Build history of the part. All positions in model axes, mm. A direction names the side the tool comes from. Give positions to 0.01 mm unless a question says otherwise; leave off trailing zeros. Write each loop counter-clockwise with the first axis right and the second up, starting at its lowest first coordinate (ties: lowest second). Pieces come first, ordered by that corner, then holes. Notation, with made-up numbers: (87.25, 70) -> (102.25, 70) arc R29 ccw to (102.25, 93) -> close; hole circle Ø8 at (22, 77.5). An arc over 180 degrees is marked (long way). One line per question, with ' | ' between items. Start each with the question number.
(1) Tool access for faces 5 (the flat face through (4.065, 0.801, 2.465)), 6 (the cylindrical face through (4.78, -3.51, 2.46)), 7 (the cylindrical face through (-0.7, 3.3, 2.5)), 8 (the cylindrical face through (-3.014, 1.518, 2.465)), 9 (the cylindrical face through (0.05, 1.65, 2.04)): list every direction of +Z, -Z, +X, -X, +Y, -Y with a clear straight run to the whole face (end or side of a thin tool).
(2) Pull direction X, two halves, no side cores. Call faces 1 (the cylindrical face through (2.19, -5.54, 2.46)), 2 (the flat face through (0, 4, 2)), 3 (the flat face through (-1.2, 2, 5)), 4 (the flat face through (-3.315, -2.486, 2.465)): released by +X, released by -X, zero draft, split by the parting line, or undercut.
(3) Band-saw the part on B-B, the plane x = -5.25. Give the cut face in (y, z), and give its area (3 significant figures).
(4) Band-saw the part on A-A, the plane y = 0. Give the cut face in (x, z) (3 decimals).
(5) Pin check, flat tips, straight feed: P1, Ø1.9, axis at x = 0, z = 3, coming from the +Y side; P2, Ø1.2, axis at y = 4.5, z = 1.5, coming from the -X side; P3, Ø2.5, axis at x = 0, y = 0, coming from the -Z side. Stop position of each tip, or through.
(6) Band-saw the part on D-D, the plane x = 6.5. Give the cut face in (y, z).
(7) Drill centre lines: probe 1 along X at (y, z) = (0, 2.3) (3 decimals); probe 2 along X at (y, z) = (3.5, 0.5); probe 3 along Z at (x, y) = (2.5, -5.25). Where is each one in solid material? Low to high. Write a range as from..to.
(8) Band-saw the part on C-C, the plane x = 3. Give the cut face in (y, z).
from build123d import *

# Parameters (mm, degrees)
SKETCH2_R                   = 6.75
GEAR_OUTSIDE_DIAMETER_DEPTH = 5
GEAR_TOOTH_CUT_DEPTH        = 6
GEAR_TEETH_COUNT            = 7
SKETCH3_R                   = 3.375
GEAR_DEDENDUM_CIRCLE_DEPTH  = 5
SKETCH5_R                   = 8
BOSS_EXTRUDE1_DEPTH         = 1
CUT_EXTRUDE1_DEPTH          = 7
CHAMFER2_SIZE               = 0.5


with BuildPart() as part:
    # Sketch2 → gear outside diameter (new body)
    with BuildSketch(Plane.XY):
        Circle(SKETCH2_R)
    extrude(amount=GEAR_OUTSIDE_DIAMETER_DEPTH)

    # Sketch1 → gear tooth cut (cut, through all)
    with BuildSketch(Plane.XY):
        with BuildLine():
            Line((0, 4.933386259), (0, 3.375))
            ThreePointArc((0, 3.375), (-0.701885443, 3.301209146), (-1.373078899, 3.083063304))
            Line((-1.373078899, 3.083063304), (-2.007089948, 4.506649523))
            ThreePointArc((-2.007089948, 4.506649523), (-2.793182164, 5.242332608), (-3.820403893, 5.564801352))
            ThreePointArc((-3.820403893, 5.564801352), (-1.403770885, 6.602418292), (1.225966143, 6.637733575))
            ThreePointArc((1.225966143, 6.637733575), (0.41879145, 5.925245269), (0, 4.933386259))
        make_face()
    gear_tooth_cut = extrude(amount=GEAR_TOOTH_CUT_DEPTH, mode=Mode.SUBTRACT)

    # gear teeth: gear tooth cut ×7 about axis
    gear_teeth_axis = Axis((0, 0, 0), (0, 0, 1))
    for i in range(1, GEAR_TEETH_COUNT):
        add(gear_tooth_cut.rotate(gear_teeth_axis, i * 360 / GEAR_TEETH_COUNT), mode=Mode.SUBTRACT)

    # Sketch3 → gear dedendum circle (add)
    with BuildSketch(Plane.XY):
        Circle(SKETCH3_R)
    extrude(amount=GEAR_DEDENDUM_CIRCLE_DEPTH)

    # Sketch5 → Boss-Extrude1 (add)
    with BuildSketch(Plane(origin=(0, 0, 0), x_dir=(-1, 0, 0), z_dir=(0, 0, -1))):
        Circle(SKETCH5_R)
    extrude(amount=BOSS_EXTRUDE1_DEPTH)

    # Sketch4 → Cut-Extrude1 (cut, through all)
    with BuildSketch(Plane.XY.offset(5)):
        with BuildLine():
            Line((-1.183215957, -1.15), (1.183215957, -1.15))
            ThreePointArc((1.183215957, -1.15), (0, 1.65), (-1.183215957, -1.15))
        make_face()
    extrude(amount=-CUT_EXTRUDE1_DEPTH, mode=Mode.SUBTRACT)

    # Chamfer2
    chamfer2_edges = [part.edges().sort_by_distance(p)[0] for p in [
        (0, 1.65, -1),
        (0, -1.15, -1),
        (0, 1.65, 5),
        (0, -1.15, 5),
    ]]
    chamfer(chamfer2_edges, length=CHAMFER2_SIZE)


solid = part.part
Results:
1) face 5: +Z, +X | face 6: +Z, -Y | face 7: +Z, +Y | face 8: +Z | face 9: +Z, -Z
2) face 1: released by +X | face 2: undercut | face 3: zero draft | face 4: released by -X
3) outline: (-6.04, -1) -> (6.04, -1) -> (6.04, 0) -> (1.23, 0) -> (1.23, 5) -> (-1.08, 5) -> (-1.08, 0) -> (-6.04, 0) -> close | area: 23.6 mm²
4) outline: (-8, -1) -> (-2.15, -1) -> (-1.65, -0.5) -> (-1.65, 4.5) -> (-2.15, 5) -> (-6.75, 5) -> (-6.75, 0) -> (-8, 0) -> close; (1.65, -0.5) -> (2.15, -1) -> (8, -1) -> (8, 0) -> (3.375, 0) -> (3.375, 5) -> (2.15, 5) -> (1.65, 4.5) -> close
5) P1: stops at y = 6.46 | P2: stops at x = -4.46 | P3: stops at z = -0.6
6) outline: (-4.66, -1) -> (4.66, -1) -> (4.66, 0) -> (-4.66, 0) -> close
7) probe 1: x = -6.75..-1.65, 1.65..3.375 | probe 2: x = -4.16..-1.56, 0..1.82 | probe 3: z = -1..0
8) outline: (-7.42, -1) -> (7.42, -1) -> (7.42, 0) -> (2.39, 0) -> (2.39, 5) -> (-2.54, 5) -> (-2.54, 0) -> (-7.42, 0) -> close
